Part model, mm, in its own coordinate system. A direction names the side the tool comes from. Round coordinates to 2 decimals unless told otherwise and drop trailing zeros. Loops run counter-clockwise (first coordinate to the right, second up) from the corner with the lowest first, then second, coordinate; pieces in that order, holes last. Notation, with made-up numbers: (-20, 20.25) -> (-6, 20.25) arc R23 ccw to (-6, 41.25) -> close; hole circle Ø3 at (-18.75, 10). An arc over 180 degrees is marked (long way). Use a Markdown table: item, result. Add a question column.
Item 1: Probe line 1 (X direction, y = 12.5, z = 3); line 2 (Z direction, x = 8, y = 4.5); line 3 (Y direction, x = 7.5, z = 2). List the from-to ranges inside material, lowest first. Write a range as [from, to].
Item 2: Two-plate mould, pull along X, no slides. Class faces 1 (the face through (16, 10, 7)), 2 (the face through (14, 7, 6)), 3 (the face through (8, 0, 11)), 4 (the face through (8, 14, 6)): pulls with the +X half, pulls with the -X half, needs draft (parallel to the pull), parting line crosses it, or undercut.
Item 3: Cut at B-B, the plane z = 6.5. List the corners of the cut face in (x, y).
Item 4: Cut at D-D, the plane y = 20. List the corners of the cut face in (x, z), plus the area to 3 significant figures.
Item 5: Cut at C-C, the plane x = 13.5. List the corners of the cut face in (y, z), plus the area to 3 significant figures.
Item 6: Which spindle directions (+Z, -Z, +X, -X, +Y, -Y) get a long thin tool onto all of the face, cutting with end or side? Do faces 5 (the face through (0.5, 15, -2)), 6 (the face through (8, 18, 1)), 7 (the face through (2, 7, 6)). Say none if no direction does.
Item 7: Flat gauge pins, fed straight in: pin 1 (3 mm diameter, centred on x = 11.5, y = 18.5, fed in from -Z); pin 2 (0.6 mm diameter, centred on x = 0.5, z = -2, fed in from -Y); pin 3 (4.5 mm diameter, centred on x = 10, z = -1.5, fed in from +Y). Where does each tip first touch, or does it go through?
Item 8: Cut at A-A, the plane y = 5. List the corners of the cut face in (x, z).
```python
from build123d import *

# Parameters (mm, degrees)
F0_W     = 16
F0_H     = 21.2
F1_DEPTH = 13.5
F2_W     = 5.9
F2_H     = 1
F3_DEPTH = 16
F4_W     = 12
F4_H     = 9.8
F5_DEPTH = 14
F6_W     = 0.5
F6_H     = 1
F7_DEPTH = 3.3


with BuildPart() as f1:
    # F0 (on Top) → F1 (new body)
    with BuildSketch(Plane.XY):
        with Locations((8, 10.6)):
            Rectangle(F0_W, F0_H)
    extrude(amount=F1_DEPTH)

    # F2 (on face) → F3 (cut, through all)
    with BuildSketch(Plane.YZ.offset(16)):
        with Locations((18.25, 0.5)):
            Rectangle(F2_W, F2_H)
    extrude(amount=-F3_DEPTH, mode=Mode.SUBTRACT)

    # F4 (on face) → F5 (cut)
    with BuildSketch(Plane.XZ):
        with Locations((8, 5.9)):
            Rectangle(F4_W, F4_H)
    extrude(amount=-F5_DEPTH, mode=Mode.SUBTRACT)

    # F6 (on face) → F7 (join)
    with BuildSketch(Plane(origin=(0, 0, 0), x_dir=(1, 0, 0), z_dir=(0, 0, -1))):
        with Locations((0.25, -14.8)):
            Rectangle(F6_W, F6_H)
        with Locations((15.75, -14.8)):
            Rectangle(F6_W, F6_H)
    extrude(amount=F7_DEPTH)


solid = f1.part
```
A:
| question | item | result |
|---|---|---|
| 1 | line 1 | x = [0, 2], [14, 16] |
| 1 | line 2 | z = [0, 1], [10.8, 13.5] |
| 1 | line 3 | y = [14, 21.2] |
| 2 | face 1 | pulls with the +X half |
| 2 | face 2 | undercut |
| 2 | face 3 | needs draft |
| 2 | face 4 | undercut |
| 3 | outline | (0, 0) -> (2, 0) -> (2, 14) -> (14, 14) -> (14, 0) -> (16, 0) -> (16, 21.2) -> (0, 21.2) -> close |
| 4 | outline | (0, 1) -> (16, 1) -> (16, 13.5) -> (0, 13.5) -> close |
| 4 | area | 200 mm^2 |
| 5 | outline | (0, 0) -> (15.3, 0) -> (15.3, 1) -> (21.2, 1) -> (21.2, 13.5) -> (0, 13.5) -> (0, 10.8) -> (14, 10.8) -> (14, 1) -> (0, 1) -> close |
| 5 | area | 143 mm^2 |
| 6 | face 5 | -Z, +Y, -Y |
| 6 | face 6 | -Z, +X, -X, +Y |
| 6 | face 7 | -Y |
| 7 | pin 1 | stops at z = 1 |
| 7 | pin 2 | stops at y = 14.3 |
| 7 | pin 3 | stops at y = 15.3 |
| 8 | outline | (0, 0) -> (16, 0) -> (16, 13.5) -> (0, 13.5) -> close; hole (2, 1) -> (14, 1) -> (14, 10.8) -> (2, 10.8) -> close |
